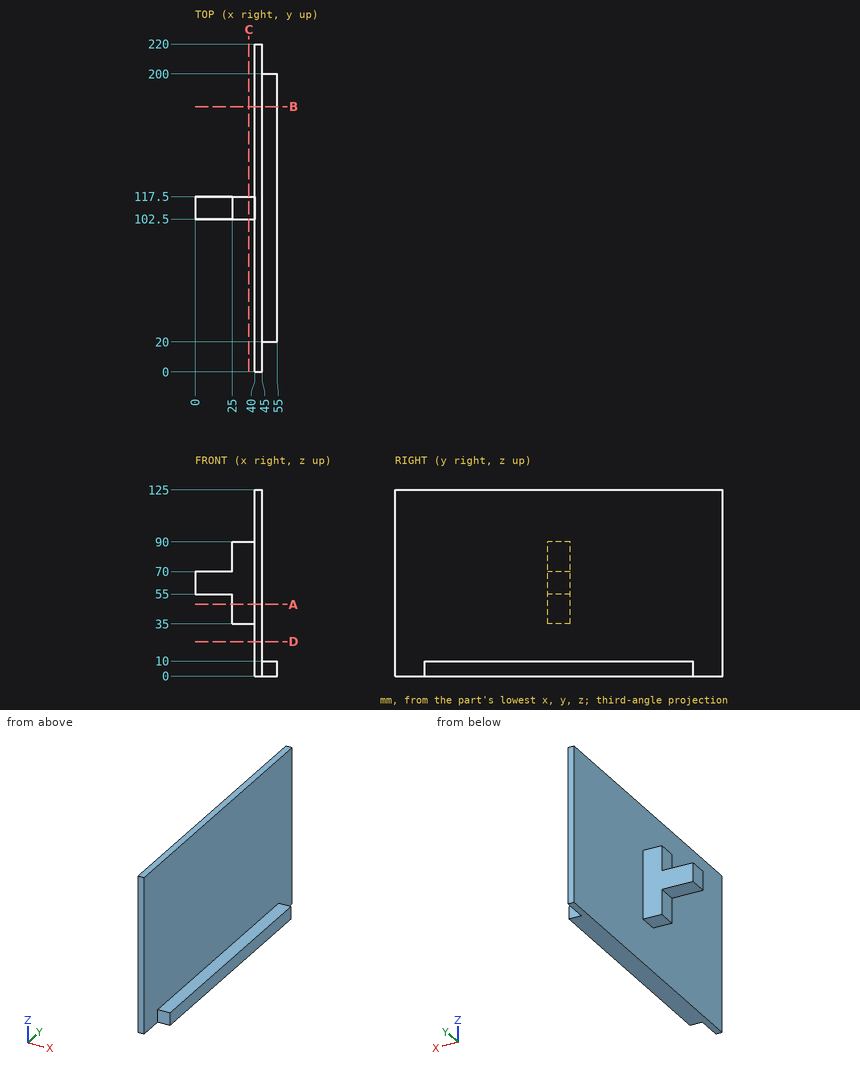
Here's the drawing with two shaded views (mm, measured from the low corner). I have some questions. Give positions to 0.01 mm unless a question says otherwise; leave off trailing zeros. Order: outer loops, then holes, each group sorted by start corner. A loop starts at its lowest first (then second) coordinate and runs counter-clockwise, first axis right, second up. Notation, with made-up numbers: M -38.75,48 L -31.75,48 A13 cw -31.75,67 Z; hole C 26.25,-11 d4. An arc over 180 degrees is marked long. Answer as a JSON object with one key per item and string values. Group by question number.
1) Suppose I cut it at B-B, the plane y = 178. Write out the boundary of the cut face in (x, z), plus the area to 3 significant figures.
2) Suppose I cut it at D-D, the plane z = 23. Write out the boundary of the cut face in (x, y).
3) Please list where these lines run through material, in increasing order: L1, parallel to X at y = 59.5, z = 65.5; L2, parallel to Z at x = 46, y = 32; L3, parallel to Z at x = 16, y = 114. Write a range as [from, to].
4) Suppose I cut it at A-A, the plane z = 48. Write out the boundary of the cut face in (x, y).
5) Suppose I cut it at C-C, the plane x = 36. Write out the boundary of the cut face in (y, z).
6) I'm going to push flat-ended pins straight in: pin 1 Ø6 at (x, y) = (18, 110.5) entering from +Z; pin 2 Ø3 at (y, z) = (67, 51) entering from -X; pin 3 Ø4.5 at (y, z) = (110, 47.5) entering from -X. Where does each tip first touch, or does it pass through?
Results found:
{
 "1": {"outline": "M 40,0 L 55,0 L 55,10 L 45,10 L 45,125 L 40,125 Z", "area": "725 mm²"},
 "2": {"outline": "M 40,0 L 45,0 L 45,220 L 40,220 Z"},
 "3": {"L1": "[40, 45]", "L2": "[0, 10]", "L3": "[55, 70]"},
 "4": {"outline": "M 25,102.5 L 40,102.5 L 40,0 L 45,0 L 45,220 L 40,220 L 40,117.5 L 25,117.5 Z"},
 "5": {"outline": "M 102.5,35 L 117.5,35 L 117.5,90 L 102.5,90 Z"},
 "6": {"pin 1": "z = 70", "pin 2": "x = 40", "pin 3": "x = 25"}
}
